Source: CAD feature listing. Evaluate the final solid. Frame: model axes, mm. Coordinates: 2 decimals unless noted, no trailing zeros. Order: outer loops, then holes, each group sorted by start corner. A loop starts at its lowest first (then second) coordinate and runs counter-clockwise, first axis right, second up.
Autodesk Inventor part; units mm, degrees
ref_plane "YZ Plane" through (0, 0, 0) normal (1, 0, 0) x (0, 1, 0)
ref_plane "XZ Plane" through (0, 0, 0) normal (0, 1, 0) x (-1, 0, 0)
ref_plane "XY Plane" through (0, 0, 0) normal (0, 0, 1) x (1, 0, 0)
sketch "Boceto1" plane through (0, 0, 0) normal (0, 0, 1) x (1, 0, 0)
  line L0 (0, 0) -> (385, 0)
  line L1 (385, 0) -> (385, 40)
  line L2 (385, 40) -> (0, 40)
  line L3 (0, 40) -> (0, 0)
  line L4 (0, 20) -> (385, 20) construction
  circle A0 centre (35, 20) radius 5
  circle A1 centre (192.5, 20) radius 5
  circle A2 centre (350, 20) radius 5
  dimension "d0" = 40
  dimension "d1" = 385
  dimension "d2" = 10
  dimension "d3" = 10
  dimension "d4" = 10
  dimension "d5" = 35
  dimension "d6" = 35
extrude "Extrusión1" add sketch "Boceto1" along normal blind 5
properties part number "Sup.Acrilico.Segur" material "Acrílico, claro"
1. Pin query (flat end, axial travel): P1, Ø3, axis at x = 67.5, y = 12.5, coming from the -Z side. Return the tip coordinate at first contact, or that it passes through.
Findings:
P1: stops at z = 0
2. Ray query, line 1 (X direction, y = 19.5, z = 1.85); line 2 (Y direction, x = 35, z = 2.5); line 3 (X direction, y = 21.5, z = 4.55). Return the intervals inside material, ascending.
Findings:
line 1: x = 0 to 30.03, 39.97 to 187.53, 197.47 to 345.03, 354.97 to 385
line 2: y = 0 to 15, 25 to 40
line 3: x = 0 to 30.23, 39.77 to 187.73, 197.27 to 345.23, 354.77 to 385
3. Section query B-B on y = 20. Return loops of the section in (x, z).
Findings:
outline: (0, 0) - (30, 0) - (30, 5) - (0, 5) - close; (40, 0) - (187.5, 0) - (187.5, 5) - (40, 5) - close; (197.5, 0) - (345, 0) - (345, 5) - (197.5, 5) - close; (355, 0) - (385, 0) - (385, 5) - (355, 5) - close
4. Draft query along X for faces 1 (the face through (31, 23, 2)), 2 (the face through (354.619, 21.915, 2.465)), 3 (the face through (190, 25, 0)). Return one class per face: released by +X, released by -X, zero draft, split by the parting line, or undercut.
Findings:
face 1: undercut
face 2: undercut
face 3: zero draft
5. Section query A-A on x = 350. Return loops of the section in (y, z).
Findings:
outline: (0, 0) - (15, 0) - (15, 5) - (0, 5) - close; (25, 0) - (40, 0) - (40, 5) - (25, 5) - close
6. Section query C-C on z = 3.5. Return loops of the section in (x, y).
Findings:
outline: (0, 0) - (385, 0) - (385, 40) - (0, 40) - close; hole circle Ø10 at (35, 20); hole circle Ø10 at (192.5, 20); hole circle Ø10 at (350, 20)
